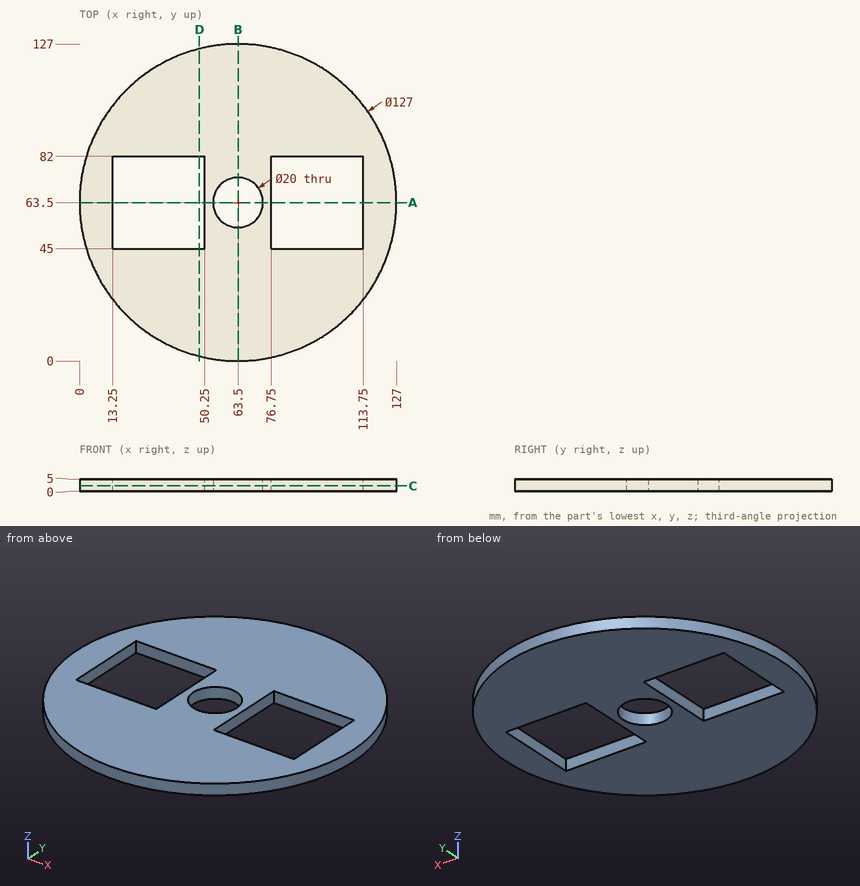
Here's the drawing with two shaded views (mm, measured from the low corner). I have some questions. Coordinates: 2 decimals unless noted, no trailing zeros. Order: outer loops, then holes, each group sorted by start corner. A loop starts at its lowest first (then second) coordinate and runs counter-clockwise, first axis right, second up.
Q1. Suppose I cut it at A-A on y = 63.5. Please give me the cut outline in (x, z), and give its area (3 significant figures).
Q2. Please list where these lines run through material, in increasing order: L1, parallel to Y at x = 63.5, z = 3.4; L2, parallel to X at y = 78.5, z = 1.15; L3, parallel to X at y = 63, z = 4.7.
Q3. Suppose I cut it at D-D on x = 48. Please give me the cut outline in (y, z), and give its area (3 significant figures).
Q4. Suppose I cut it at B-B on x = 63.5. Please give me the cut outline in (y, z), and give its area (3 significant figures).
Q5. Will these pins go through, and if not, where does the flat tip stop? pin 1 (2 mm diameter, centred on x = 87, z = 3.5, fed in from +Y); pin 2 (1.5 mm diameter, centred on x = 103, z = 3, fed in from +Y); pin 3 (2.5 mm diameter, centred on x = 25, z = 1.5, fed in from +Y); pin 4 (1 mm diameter, centred on x = 103, y = 81, fed in from +Z).
Q6. Suppose I cut it at C-C on z = 2.2. Please give me the cut outline in (x, y).
Answer:
1. outline: (0, 0) - (13.25, 0) - (13.25, 5) - (0, 5) - close; (50.25, 0) - (53.5, 0) - (53.5, 5) - (50.25, 5) - close; (73.5, 0) - (76.75, 0) - (76.75, 5) - (73.5, 5) - close; (113.75, 0) - (127, 0) - (127, 5) - (113.75, 5) - close
1. area: 165 mm2
2. L1: y = 0 to 53.5, 73.5 to 127
2. L2: x = 1.8 to 13.25, 50.25 to 76.75, 113.75 to 125.2
2. L3: x = 0 to 13.25, 50.25 to 53.51, 73.49 to 76.75, 113.75 to 127
3. outline: (1.92, 0) - (45, 0) - (45, 5) - (1.92, 5) - close; (82, 0) - (125.08, 0) - (125.08, 5) - (82, 5) - close
3. area: 431 mm2
4. outline: (0, 0) - (53.5, 0) - (53.5, 5) - (0, 5) - close; (73.5, 0) - (127, 0) - (127, 5) - (73.5, 5) - close
4. area: 535 mm2
5. pin 1: stops at y = 122.88
5. pin 2: stops at y = 113.81
5. pin 3: stops at y = 114.93
5. pin 4: passes through
6. outline: circle Ø127 at (63.5, 63.5); hole (13.25, 45) - (50.25, 45) - (50.25, 82) - (13.25, 82) - close; hole circle Ø20 at (63.5, 63.5); hole (76.75, 45) - (113.75, 45) - (113.75, 82) - (76.75, 82) - close
